Read the model definition and answer for the solid it produces. Units are mm, in the model's axes. A direction names the side the tool comes from. Round coordinates to 2 decimals unless told otherwise and drop trailing zeros. Order: outer loops, then holes, each group sorted by start corner. A loop starts at its lowest first (then second) coordinate and runs counter-clockwise, first axis right, second up.
from build123d import *

# Parameters (mm, degrees)
F2_SIZE = 0.25


with BuildPart() as f1:
    # F0 (on Front) → F1 (revolve)
    with BuildSketch(Plane.XZ):
        Polygon((80.8070451021, 45.6162330286), (98.8070451021, 45.6162330286), (98.8070451021, 46.8662330286), (93.8070451021, 46.8662330286), (93.8070451021, 46.6162330286), (92.8070451021, 46.6162330286), (92.8070451021, 46.8662330286), (80.8070451021, 46.8662330286), align=None)
        Polygon((62.8070451021, 45.6162330286), (80.8070451021, 45.6162330286), (80.8070451021, 46.8662330286), (68.8070451021, 46.8662330286), (68.8070451021, 46.6162330286), (67.8070451021, 46.6162330286), (67.8070451021, 46.8662330286), (62.8070451021, 46.8662330286), align=None)
    revolve(axis=Axis((89.8070451021, 0, 45.6162330286), (1, 0, 0)))

    # F2
    f2_edges = [f1.edges().sort_by_distance(p)[0] for p in [
        (98.807045, 0, 44.366233),
        (62.807045, 0, 44.366233),
    ]]
    chamfer(f2_edges, length=F2_SIZE)


solid = f1.part
Q1. Flat-ended cylindrical pins translate along their axes: pin 1 (1 mm diameter, centred on x = 67.5, z = 45, fed in from -Y); pin 2 (1 mm diameter, centred on x = 78, z = 44.5, fed in from +Y). Find the tip coordinate at first contact, or state that the pin passes through.
Outcome:
pin 1: stops at y = -1.24
pin 2: stops at y = 1.09
Q2. For a pull along X with two mould halves and no side action, classify faces 3 (the face through (68.3, -0.044, 44.617)), 4 (the face through (62.807, 0, 46)), 5 (the face through (98.807, 0, 46)) as released by +X, released by -X, zero draft, split by the parting line, or undercut.
Outcome:
face 3: undercut
face 4: released by -X
face 5: released by +X
Q3. Straight lines are drawn through the part: probe 1 along X at (y, z) = (-0.8, 46.4); probe 2 along Z at (x, y) = (71.5, -0.1); probe 3 along Y at (x, z) = (65, 45.5). For each, find the intervals that lie inside material, in ascending order.
Outcome:
probe 1: x = 62.93 to 67.81, 68.81 to 92.81, 93.81 to 98.69
probe 2: z = 44.37 to 46.86
probe 3: y = -1.24 to 1.24
Q4. A cutting plane is placed at A-A, the plane x = 91. Give the vertices of the cut face in (y, z), plus the area to 3 significant figures.
Outcome:
outline: circle Ø2.5 at (0, 45.62)
area: 4.91 mm2
Q5. For faces 1 (the face through (96.1, -0.4, 46.8)), 2 (the face through (93.3, -0.044, 44.617)), determine the directions among +Z, -Z, +X, -X, +Y, -Y from which every point of the face is accessible in a straight line to the end or side of a thin tool.
Outcome:
face 1: +X, -X
face 2: none
